Read the model definition and answer for the solid it produces. Units are mm, in the model's axes. A direction names the side the tool comes from. Coordinates: 2 decimals unless noted, no trailing zeros. Loops run counter-clockwise (first coordinate to the right, second up) from the corner with the lowest first, then second, coordinate; pieces in that order, holes last. Notation, with made-up numbers: M 59,-4 L 102,-4 A29 ccw 102,20 Z; hole C 2.25,8 d9. An arc over 180 degrees is marked long. Use one line per item in the form item = value. Start each with the question number.
1. The part is cut by section D-D (x = -9.25). Give the vertices of the cut face in (y, z), plus the area to 3 significant figures.
2. For a pull along Y with two mould halves and no side action, classify faces 1 (the flat face through (0, 8.5, 18)), 2 (the cylindrical face through (-5.5, 4.32, 10.07)), 3 (the cylindrical face through (0.54, 2.44, 10.14)), 4 (the conical face through (6.74, 6.745, 10.011)) as released by +Y, released by -Y, zero draft, split by the parting line, or undercut.
3. The part is cut by section B-B (z = 17.75). Give the vertices of the cut face in (x, y).
4. A tool of negligible diameter and unlimited length cuts with its end or side. For faces 5 (the flat face through (0, -8.5, 18)), 6 (the cylindrical face through (-4.5, -11.9, 9.9)), 7 (the flat face through (0, 11, 15)), from which of +Z, -Z, +X, -X, +Y, -Y can it reach the whole face along a straight path? Write none if from no direction.
5. The part is cut by section A-A (x = 0). Give the vertices of the cut face in (y, z), plus the area to 3 significant figures.
6. Flat-ended cylindrical pins translate along their axes: pin 1 (12 mm diameter, centred on x = -3, z = 8.5, fed in from -Y); pin 2 (6 mm diameter, centred on x = -1, y = 12, fed in from +Z); pin 3 (5.5 mm diameter, centred on x = 4.5, z = 18, fed in from -Y); pin 4 (1 mm diameter, centred on x = -4.5, z = 5, fed in from +Y). Find the tip coordinate at first contact, or state that the pin passes through.
7. Find the intervals of material crossed by probe 1 along X at (y, z) = (-8.5, 10); probe 2 along Y at (x, z) = (-7, 16.25); probe 3 along Z at (x, y) = (7, -11.65), in increasing order. Write a range as [from, to].
8. The part is cut by section C-C (y = -7.5). Give the vertices of the cut face in (x, z).
from build123d import *

# Parameters (mm, degrees)
F0_R           = 14
F0_R_2         = 3
F0_R_3         = 1
F1_DEPTH       = 20
F2_D           = 6
F5_D           = 3
F5_DEPTH       = 20
F5_CBORE_D     = 5
F5_CBORE_DEPTH = 3
F5_TIP         = 0.9012909285
F7_DEPTH       = 5
F8_D           = 5


with BuildPart() as f1:
    # F0 (on Top) → F1 (new body)
    with BuildSketch(Plane.XY):
        Circle(F0_R)
        with Locations((-7, 0)):
            Circle(F0_R_2, mode=Mode.SUBTRACT)
        Circle(F0_R_2, mode=Mode.SUBTRACT)
        with Locations((0, 5)):
            Circle(F0_R_3, mode=Mode.SUBTRACT)
        with Locations((7, 0)):
            Circle(F0_R_2, mode=Mode.SUBTRACT)
        with Locations((-7, 0)):
            Circle(F0_R_2)
        Circle(F0_R_2)
        with Locations((7, 0)):
            Circle(F0_R_2)
        with Locations((0, 5)):
            Circle(F0_R_3)
    extrude(amount=F1_DEPTH)

    # F2 (through all)
    with Locations(Plane(origin=(0, 0, 0), x_dir=(1, 0, 0), z_dir=(0, 0, -1))):
        with Locations((-7, 0), (7, 0)):
            Hole(F2_D / 2)

    # F5
    with Locations(Plane.XZ.offset(14)):
        with Locations((-7, 10), (7, 10)):
            CounterBoreHole(F5_D / 2, F5_CBORE_D / 2, F5_CBORE_DEPTH, depth=F5_DEPTH)
            with Locations((0, 0, -(F5_DEPTH + F5_TIP / 2))):  # 118° drill point
                Cone(0, F5_D / 2, F5_TIP, mode=Mode.SUBTRACT)

    # F6 (on face) → F7 (cut)
    with BuildSketch(Plane.XY.offset(20)):
        with BuildLine():
            Line((-11.1242977306, 8.5), (11.1242977306, 8.5))
            ThreePointArc((11.1242977306, 8.5), (0, 14), (-11.1242977306, 8.5))
        make_face()
        with BuildLine():
            ThreePointArc((-11.1242977306, -8.5), (0, -14), (11.1242977306, -8.5))
            Line((11.1242977306, -8.5), (-11.1242977306, -8.5))
        make_face()
    extrude(amount=-F7_DEPTH, mode=Mode.SUBTRACT)

    # F8 (through all)
    with Locations(Plane(origin=(0, 0, 0), x_dir=(1, 0, 0), z_dir=(0, 0, -1))):
        with Locations((0, 0)):
            Hole(F8_D / 2)


solid = f1.part
Computed values:
q1.outline = M -10.51,0 L -1.98,0 L -1.98,20 L -8.5,20 L -8.5,15 L -10.51,15 Z; M 1.98,0 L 10.51,0 L 10.51,15 L 8.5,15 L 8.5,20 L 1.98,20 Z
q1.area = 321 mm²
q2.face_1 = released by +Y
q2.face_2 = zero draft
q2.face_3 = undercut
q2.face_4 = released by -Y
q3.outline = M -11.12,-8.5 L 11.12,-8.5 A14 ccw 11.12,8.5 L -11.12,8.5 A14 ccw Z; hole C -7,0 d6; hole C 0,0 d5; hole C 7,0 d6
q4.face_5 = +Z, +X, -X, -Y
q4.face_6 = -Y
q4.face_7 = +Z, +X, -X, +Y
q5.outline = M -14,0 L -2.5,0 L -2.5,20 L -8.5,20 L -8.5,15 L -14,15 Z; M 2.5,0 L 14,0 L 14,15 L 8.5,15 L 8.5,20 L 2.5,20 Z
q5.area = 405 mm²
q6.pin_1 = -14
q6.pin_2 = 15
q6.pin_3 = -8.5
q6.pin_4 = 13.42
q7.probe_1 = [-11.12, -8.5], [-5.5, 5.5], [8.5, 11.12]
q7.probe_2 = [-8.5, -3], [3, 8.5]
q7.probe_3 = [0, 7.5], [12.5, 15]
q8.outline = M -11.82,0 L 11.82,0 L 11.82,20 L -11.82,20 Z; hole C -7,10 d3; hole C 7,10 d3
